Autodesk Inventor part; units mm, degrees
ref_plane "YZ Plane" through (0, 0, 0) normal (1, 0, 0) x (0, 1, 0)
ref_plane "XZ Plane" through (0, 0, 0) normal (0, 1, 0) x (-1, 0, 0)
ref_plane "XY Plane" through (0, 0, 0) normal (0, 0, 1) x (1, 0, 0)
sketch "Sketch1" plane through (0, 0, 0) normal (1, 0, 0) x (0, 1, 0)
  line L0 (0, 0) -> (50.8, 0)
  line L1 (50.8, 0) -> (50.8, -101.6)
  line L2 (50.8, -101.6) -> (0, -101.6)
  line L3 (0, -101.6) -> (0, 0)
  dimension "d0" = 101.6
  dimension "d1" = 50.8
extrude "Extrusion1" add sketch "Sketch1" along normal blind 400
shell "Shell1" thickness 6.35 removed faces 2 at (0, 16.9333, -33.8667) at (400, 16.9333, -33.8667)
sketch "Sketch2" plane through (0, 50.8, 0) normal (0, 1, 0) x (1, 0, 0)
  circle A0 centre (395, 70.8) radius 2
  circle A1 centre (395, 30.8) radius 2
  circle A2 centre (342, 70.8) radius 2
  circle A3 centre (342, 30.8) radius 2
  line L0 (395, 70.8) -> (342, 70.8) construction
  line L1 (342, 70.8) -> (342, 30.8) construction
  line L2 (342, 30.8) -> (395, 30.8) construction
  line L3 (395, 30.8) -> (395, 70.8) construction
  line L4 (400, 101.6) -> (400, 0)
  line L5 (337, 101.6) -> (337, 0)
  line L6 (337, 0) -> (400, 0)
  line L7 (400, 101.6) -> (337, 101.6)
  point P0 (368.5, 0)
  point P1 (368.5, 30.8)
  point P2 (395, 50.8)
  point P3 (400, 50.8)
  dimension "d5" = 4
  dimension "d6" = 63
  dimension "d7" = 40
  dimension "d8" = 53
extrude "Extrusion2" cut sketch "Sketch2" against normal up to surface (6.35 mm away) contours A0 | A1 | A2 | A3
sketch "Sketch3" plane through (0, 0, 0) normal (0, 0, 1) x (1, 0, 0)
  line L0 (397, 44.45) -> (393, 44.45) construction
  line L1 (344, 44.45) -> (340, 44.45) construction
  circle A0 centre (368.5, 25.4) radius 19 construction
  line L2 (400, 50.8) -> (400, 0) construction
  line L3 (393, 44.45) -> (368.5, 25.4) construction
  line L4 (368.5, 25.4) -> (344, 44.45) construction
  circle A1 centre (355.065, 11.965) radius 2
  circle A2 centre (381.935, 11.965) radius 2
  circle A3 centre (381.935, 38.835) radius 2
  circle A4 centre (387.5, 25.4) radius 2
  circle A5 centre (355.065, 38.835) radius 2
  circle A6 centre (349.5, 25.4) radius 2
  line L5 (349.5, 25.4) -> (368.5, 25.4) construction
  line L6 (355.065, 11.965) -> (368.5, 25.4) construction
  circle A7 centre (368.5, 25.4) radius 14
  point P0 (0, 0)
  point P1 (400, 25.4)
  point P2 (400, 25.4)
  dimension "d11" = 38
  dimension "d12" = 4
  dimension "d13" = 45
  dimension "d14" = 28
extrude "Extrusion3" cut sketch "Sketch3" against normal up to surface (6.35 mm away)
sketch "Sketch4" plane through (0, 0, -101.6) normal (0, 0, -1) x (-1, 0, 0)
  circle A0 centre (-368.5, 25.4) radius 14 construction
  circle A1 centre (-368.5, 25.4) radius 8.25
  point P0 (0, 0)
  dimension "d17" = 16.5
extrude "Extrusion4" cut sketch "Sketch4" against normal up to surface (6.35 mm away)
sketch "Sketch5" plane through (0, 0, -101.6) normal (0, -1, 0) x (1, 0, 0)
  circle A0 centre (342, 30.8) radius 2
  circle A1 centre (342, 70.8) radius 2
  circle A2 centre (342, 30.8) radius 5
  circle A3 centre (342, 70.8) radius 5
  point P0 (0, 101.6)
  dimension "d20" = 10
extrude "Extrusion5" cut sketch "Sketch5" against normal up to surface (6.35 mm away) contours A0 | A1 | A2 | A3
properties part number "VERTICALTUBE"
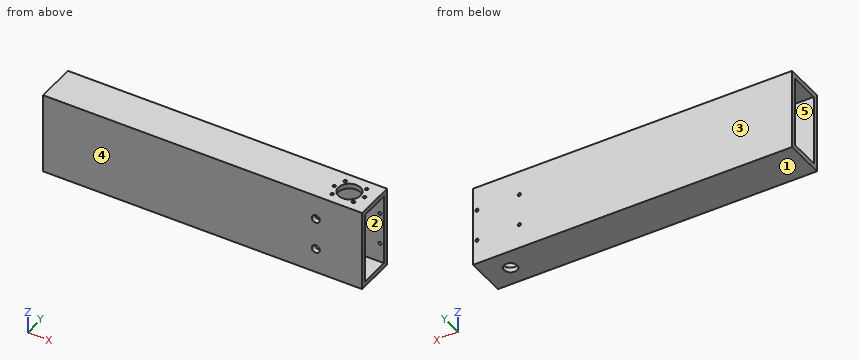
Can you work these out from the model? Positions are in its coordinate system, mm. Face numbers are marked on the shaded views. A direction names the side the tool comes from. Coordinates: 2 decimals unless noted, no trailing zeros. Loops run counter-clockwise (first coordinate to the right, second up) from the corner with the lowest first, then second, coordinate; pieces in that order, holes last.
1) Thinking about a two-plate mould opening in Y: for the marked faces 1, 2 and 3, which applies, pulls with the +Y half, pulls with the -Y half, needs draft (parallel to the pull), parting line crosses it, or undercut?
2) For pin 1 (1.5 mm diameter, centred on x = 120.5, z = -90, fed in from -Y); pin 2 (8 mm diameter, centred on y = 11, z = -51, fed in from +X); pin 3 (3 mm diameter, centred on x = 395, z = -30.8, fed in from +Y); pin 4 (3 mm diameter, centred on x = 355.065, y = 11.965, fed in from +Z), each with a flat end and sliding along its axis, tell me the tip position at first contact or that it passes through.
3) Imagine slicing it at B-B on x = 193. List the corners of the cut face in (y, z) for me.
4) Which directions (+Z, -Z, +X, -X, +Y, -Y) give clear straight access to the entire face, cutting with the end or side of a thin tool? Please do the marked faces 4 and 5.
5) I need wall thicknesses on probe 1 along Z at (x, y) = (342, 49); probe 2 along X at (y, z) = (48.5, -70.8); probe 3 along X at (y, z) = (2, -30). Which ranges of each line are inside material? Lowest first, please.
6) Imagine slicing it at A-A on z = -19. List the corners of the cut face in (x, y) for me.
Completed:
1. face 1: needs draft
1. face 2: undercut
1. face 3: pulls with the +Y half
2. pin 1: stops at y = 0
2. pin 2: passes through
2. pin 3: stops at y = 6.35
2. pin 4: stops at z = -95.25
3. outline: (0, -101.6) - (50.8, -101.6) - (50.8, 0) - (0, 0) - close; hole (6.35, -95.25) - (44.45, -95.25) - (44.45, -6.35) - (6.35, -6.35) - close
4. face 4: +Z, -Z, +X, -X, -Y
4. face 5: +X, -X
5. probe 1: z = -101.6 to -72.8, -68.8 to -32.8, -28.8 to 0
5. probe 2: x = 0 to 340, 344 to 393, 397 to 400
5. probe 3: x = 0 to 337.06, 346.94 to 400
6. outline: (0, 0) - (400, 0) - (400, 6.35) - (0, 6.35) - close; (0, 44.45) - (400, 44.45) - (400, 50.8) - (0, 50.8) - close
